Check sheet for the modelled part. Datum: model origin and axes. Units: mm. Round coordinates to 2 decimals unless told otherwise and drop trailing zeros. Write each loop counter-clockwise with the first axis right and the second up, starting at its lowest first coordinate (ties: lowest second). Pieces come first, ordered by that corner, then holes. Notation, with made-up numbers: M -37.5,3.5 L -4.5,3.5 A18 ccw -4.5,33.5 Z; hole C 13,-39.5 d2. An arc over 180 degrees is marked long. Put each result on its own line as item: value.
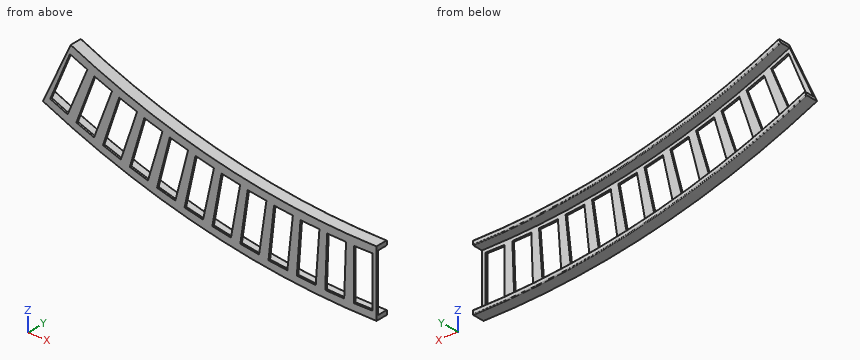
```python
from build123d import *

# Parameters (mm, degrees)
REVOLVE1_ANGLE     = 25
SKETCH4_W          = 15
SKETCH4_H          = 40
CUT_EXTRUDE3_DEPTH = 10


with BuildPart() as part:
    # Sketch1 → Revolve1 (revolve)
    with BuildSketch(Plane(origin=(0, 0, 0), x_dir=(0, 0, -1), z_dir=(1, 0, 0))):
        with BuildLine():
            ThreePointArc((22.5, 9.4), (22.675735931, 9.824264069), (23.1, 10))
            Line((23.1, 10), (25.4, 10))
            ThreePointArc((25.4, 10), (25.824264069, 9.824264069), (26, 9.4))
            Line((26, 9.4), (26, 0))
            Line((26, 0), (-26, 0))
            Line((-26, 0), (-26, 9.4))
            ThreePointArc((-26, 9.4), (-25.824264069, 9.824264069), (-25.4, 10))
            Line((-25.4, 10), (-23.1, 10))
            ThreePointArc((-23.1, 10), (-22.675735931, 9.824264069), (-22.5, 9.4))
            Line((-22.5, 9.4), (-22.5, 1.5))
            Line((-22.5, 1.5), (22.5, 1.5))
            Line((22.5, 1.5), (22.5, 9.4))
        make_face()
    revolve(axis=Axis((0, -3.326119583, 600), (0, 1, 0)), revolution_arc=REVOLVE1_ANGLE)

    # Sketch4 → Cut-Extrude3 (cut)
    with BuildSketch(Plane(origin=(0, 0, 0), x_dir=(1, 0, 0), z_dir=(0, 1, 0))):
        with Locations((-10.5, 0)):
            Rectangle(SKETCH4_W, SKETCH4_H)
        Polygon((-40.608807593, 18.930468426), (-39.149401653, -21.042899387), (-24.159388723, -20.495622159), (-25.618794663, 19.477745654), align=None)
        Polygon((-63.163540118, 17.036763248), (-60.246671595, -22.856743467), (-45.286606577, -21.762917771), (-48.2034751, 18.130588944), align=None)
        Polygon((-85.634163481, 14.321406142), (-81.263716507, -25.439116908), (-66.353520363, -23.800199292), (-70.723967338, 15.960323758), align=None)
        Polygon((-107.990755592, 10.788012904), (-102.172549893, -28.786580998), (-87.33207718, -26.60475386), (-93.150282879, 12.969840041), align=None)
        Polygon((-130.203546201, 6.441288631), (-122.945329355, -32.894678221), (-108.194341785, -30.172846904), (-115.452558632, 9.163119949), align=None)
        Polygon((-152.24295655, 1.287021464), (-143.554393666, -37.757938198), (-128.912533793, -34.499727117), (-137.601096677, 4.545232545), align=None)
        Polygon((-174.079638754, -4.667925128), (-163.972299604, -43.369884966), (-149.459064664, -39.579632785), (-159.566403814, -0.877672947), align=None)
        Polygon((-195.684514881, -11.415621482), (-184.171858492, -49.723045604), (-169.806574446, -45.405799458), (-181.319230835, -7.098375336), align=None)
        Polygon((-217.028815677, -18.947082302), (-204.126172411, -56.808960184), (-189.927968205, -51.970468959), (-202.830611472, -14.108591077), align=None)
        Polygon((-238.084118872, -27.252278624), (-223.808670008, -64.618193035), (-209.796452104, -59.264899711), (-224.071900968, -21.8989853), align=None)
        Polygon((-258.822387025, -36.320151172), (-243.193141886, -73.14034531), (-229.385569084, -67.279378383), (-245.014814224, -30.459184245), align=None)
    extrude(amount=CUT_EXTRUDE3_DEPTH, mode=Mode.SUBTRACT)


solid = part.part
```
1. Cross-section at A-A (y = 7.75). Enter the section's corners in (x, z).
Computed values:
outline: M -264.56,32.65 A626 ccw 0,-26 L 0,-22.5 A622.5 cw -263.08,35.82 Z; M -244.06,76.61 A577.5 ccw 0,22.5 L 0,26 A574 cw -242.58,79.78 Z
2. Scan lines: probe 1 along Y at (x, z) = (-44.5, 9); probe 2 along Z at (x, y) = (-17, 7.75); probe 3 along Z at (x, y) = (-176, 8). Record each from-to range of solid material in increasing order.
Computed values:
probe 1: y = 0 to 1.5
probe 2: z = -25.77 to -22.27, 22.75 to 26.25
probe 3: z = -0.75 to 2.9, 49.97 to 53.65
3. Depth check by flat-ended pin: pin 1 Ø12 at (x, z) = (-75.5, 14) entering from +Y; pin 2 Ø1 at (x, y) = (-94.5, 7) entering from -Z. Enter the tip coordinate at first touch or a pass-through.
Computed values:
pin 1: passes through
pin 2: stops at z = -18.9
